Design review of the part built by this model. Coordinates are the model's own, in mm. Face numbers are marked on the shaded views. A direction names the side the tool comes from. Round coordinates to 2 decimals unless told otherwise and drop trailing zeros. Order: outer loops, then holes, each group sorted by start corner. A loop starts at its lowest first (then second) coordinate and runs counter-clockwise, first axis right, second up. Notation, with made-up numbers: M 45.25,73 L 49.25,73 A19 cw 49.25,109 Z; hole C 87,26 d4. An arc over 180 degrees is marked long. Use a Markdown table: item, result. Add a question column.
(1) The part is to be moulded in two halves that separate along X. For the marked faces 1, 2, 3 and 4, say which applies: released by +X, released by -X, zero draft, split by the parting line, or undercut.
(2) Take a section at A-A (z = 7.5). Write out the cut boundary in (x, y).
(3) Take a section at B-B (x = -20.5). Write out the cut boundary in (y, z).
(4) For pin 1 (12 mm diameter, centred on x = -11.5, z = 1.5, fed in from +Y), flat-tipped, find the tip position at first contact; note if it passes through.
(5) Machinability: for the marked faces 5 and 6, which of the approach directions +Z, -Z, +X, -X, +Y, -Y give a long, thin tool a straight path to every point of the face, cutting with its end or side? Answer none if there is none.
(6) Take a section at D-D (x = -38.5). Write out the cut boundary in (y, z).
(7) Take a section at C-C (y = 2). Count the separate pieces of the cut face and the enclosed holes in it, then the cut area to 3 significant figures.
(8) To check wall thickness, follow probe 1 along X at (y, z) = (2, -11); probe 2 along Z at (x, y) = (-24, 4); probe 3 along X at (y, z) = (-0.5, 5). State the ranges of each line that lie inside material, in increasing order. Write a range as from..to.
```python
from build123d import *

# Parameters (mm, degrees)
F0_W          = 50
F0_H          = 50
F0_R          = 3
F0_R_2        = 2.5
F1_DEPTH      = 5
F0_W_2        = 4.763
F0_H_2        = 4.763
F2_DEPTH      = 5
F3_DEPTH      = 15
F3_DEPTH_BACK = 5


with BuildPart() as f1:
    # F0 (on Front) → F1 (new body, symmetric)
    with BuildSketch(Plane.XZ):
        with Locations((-17.8228546229, -1.0937498882)):
            Rectangle(F0_W, F0_H)
        with Locations((-37.8228546229, -21.0937498882)):
            Circle(F0_R, mode=Mode.SUBTRACT)
        with Locations((2.1771453771, -21.0937498882)):
            Circle(F0_R_2, mode=Mode.SUBTRACT)
        Polygon((-37.6238546229, 8.4166441185), (-32.8608546229, 8.4166441185), (-16.6755962394, 8.4166441185), (-16.6755962394, 14.7900106385), (-11.9125962394, 14.7900106385), (-11.9125962394, 8.4166441185), (-2.5272074943, 8.4166441185), (-2.5272074943, -12.8520363942), (-13.7815852112, -12.8520363942), (-19.5766687393, -12.8520363942), (-19.5766687393, -10.0679453462), (-27.1787202845, -10.0679453462), (-27.1787202845, -9.4257498882), (-31.0388546229, -9.4257498882), (-31.0388546229, -14.1887498882), (-35.8018546229, -14.1887498882), (-35.8018546229, -9.4257498882), (-35.8018546229, -5.3049453462), (-27.1787202845, -5.3049453462), (-14.8136687393, -5.3049453462), (-14.8136687393, -8.8673923165), (-7.2902074943, -8.8673923165), (-7.2902074943, -4.3980097398), (-14.436878264, -4.3980097398), (-14.436878264, 0.3649902602), (-8.9991306886, 0.3649902602), (-8.9991306886, 3.6536441185), (-16.6755962394, 3.6536441185), (-32.8608546229, 3.6536441185), (-37.6238546229, 3.6536441185), align=None, mode=Mode.SUBTRACT)
        with Locations((-37.8228546229, 18.9062501118)):
            Circle(F0_R_2, mode=Mode.SUBTRACT)
        with Locations((2.1771453771, 18.9062501118)):
            Circle(F0_R, mode=Mode.SUBTRACT)
    extrude(amount=F1_DEPTH, both=True)

    # F0 (on Front) → F2 (join)
    with BuildSketch(Plane.XZ):
        Polygon((-16.6755962394, 8.4166441185), (-32.8608546229, 8.4166441185), (-32.8608546229, 3.6536441185), (-16.6755962394, 3.6536441185), (-8.9991306886, 3.6536441185), (-8.9991306886, 0.3649902602), (-14.436878264, 0.3649902602), (-14.436878264, -4.3980097398), (-7.2902074943, -4.3980097398), (-7.2902074943, -8.8673923165), (-14.8136687393, -8.8673923165), (-14.8136687393, -5.3049453462), (-27.1787202845, -5.3049453462), (-35.8018546229, -5.3049453462), (-35.8018546229, -9.4257498882), (-31.0388546229, -9.4257498882), (-27.1787202845, -9.4257498882), (-27.1787202845, -10.0679453462), (-19.5766687393, -10.0679453462), (-19.5766687393, -12.8520363942), (-13.7815852112, -12.8520363942), (-2.5272074943, -12.8520363942), (-2.5272074943, 8.4166441185), (-11.9125962394, 8.4166441185), (-11.9125962394, 14.7900106385), (-16.6755962394, 14.7900106385), align=None)
        with Locations((-33.4203546229, -11.8072498882)):
            Rectangle(F0_W_2, F0_H_2)
    extrude(amount=F2_DEPTH)

    # F0 (on Front) → F3 (join, two sides)
    with BuildSketch(Plane.XZ) as f3_sk:
        with Locations((2.1771453771, -21.0937498882)):
            Circle(F0_R_2)
        with Locations((-37.8228546229, 18.9062501118)):
            Circle(F0_R_2)
    extrude(amount=-F3_DEPTH)
    extrude(f3_sk.sketch, amount=F3_DEPTH_BACK)


solid = f1.part
```
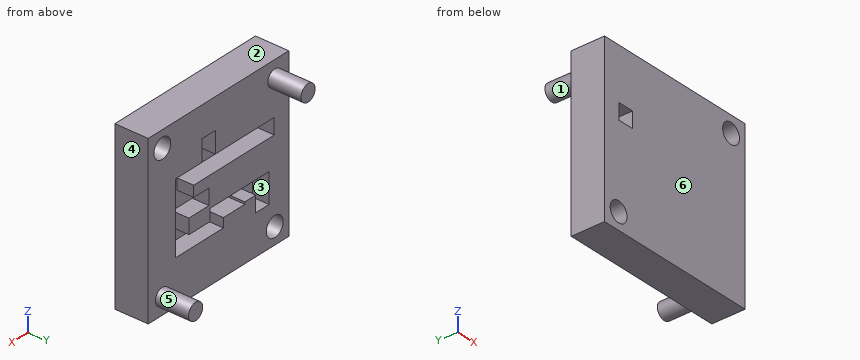
Verdict:
| question | item | result |
|---|---|---|
| 1 | face 1 | split by the parting line |
| 1 | face 2 | zero draft |
| 1 | face 3 | undercut |
| 1 | face 4 | released by +X |
| 2 | outline | M -42.82,-5 L -37.62,-5 L -37.62,5 L -42.82,5 Z; M -32.86,-5 L 7.18,-5 L 7.18,5 L -2.53,5 L -2.53,0 L -32.86,0 Z |
| 3 | outline | M -5,-26.09 L 5,-26.09 L 5,-10.07 L 0,-10.07 L 0,-5.3 L 5,-5.3 L 5,3.65 L 0,3.65 L 0,8.42 L 5,8.42 L 5,23.91 L -5,23.91 Z |
| 4 | pin 1 | stops at y = 5 |
| 5 | face 5 | +Y |
| 5 | face 6 | +Z, -Z, +X, -X, -Y |
| 6 | outline | M -5,-26.09 L 5,-26.09 L 5,-24.02 L -5,-24.02 Z; M -5,-18.17 L 5,-18.17 L 5,16.5 L 15,16.5 L 15,21.31 L 5,21.31 L 5,23.91 L -5,23.91 Z |
| 7 | separate pieces | 1 |
| 7 | enclosed holes | 3 |
| 7 | area | 1,970 mm^2 |
| 8 | probe 1 | x = -42.82..-35.8, -31.04..-19.58, -2.53..7.18 |
| 8 | probe 2 | z = -26.09..-10.07, -5.3..3.65, 8.42..23.91 |
| 8 | probe 3 | x = -42.82..-37.62, -32.86..7.18 |
